```python
from build123d import *

# Parameters (mm, degrees)
F1_DEPTH = 30
F2_R     = 3
F3_DEPTH = 60.001
F5_DEPTH = 30.001


with BuildPart() as f1:
    # F0 (on Front) → F1 (new body)
    with BuildSketch(Plane.XZ):
        Polygon((0, 30), (0, 0), (60, 0), (60, 3), (3, 3), (3, 30), align=None)
    extrude(amount=F1_DEPTH)

    # F2 (on face) → F3 (cut, through all)
    with BuildSketch(Plane(origin=(0, 0, 0), x_dir=(0, -1, 0), z_dir=(-1, 0, 0))):
        with Locations((15, 15)):
            Circle(F2_R)
    extrude(amount=-F3_DEPTH, mode=Mode.SUBTRACT)

    # F4 (on face) → F5 (cut, through all)
    with BuildSketch(Plane(origin=(0, 0, 0), x_dir=(1, 0, 0), z_dir=(0, 0, -1))):
        with BuildLine():
            Line((52, 18), (48.109772, 18))
            ThreePointArc((48.109772, 18), (38, 15), (48.109772, 12))
            Line((48.109772, 12), (52, 12))
            ThreePointArc((52, 12), (55, 15), (52, 18))
        make_face()
    extrude(amount=-F5_DEPTH, mode=Mode.SUBTRACT)


solid = f1.part
```
Input: part model. Units: mm. Frame: model coordinates. A direction names the side the tool comes from. Round coordinates to 2 decimals unless told otherwise and drop trailing zeros. Loops run counter-clockwise (first coordinate to the right, second up) from the corner with the lowest first, then second, coordinate; pieces in that order, holes last. Notation, with made-up numbers: (74.25, 23.5) -> (90.25, 23.5) arc R12 ccw to (90.25, 28.5) -> close; hole circle Ø10 at (64, 65). An arc over 180 degrees is marked (long way). Use one line per item in the form item = value. Start each with the question number.
Item 1: Section query C-C on x = 43.5. Return the cut outline in (y, z), then the cut area to 3 significant figures.
Item 2: Section query D-D on y = -10.75. Return the cut outline in (x, z), then the cut area to 3 significant figures.
Item 3: Contact query for a flat-ended pin moving along its axis: pin 1 Ø1.5 at (x, y) = (28, -11.5) entering from +Z. Output: stop coordinate, or through.
Item 4: Section query B-B on y = -15. Return the cut outline in (x, z), then the cut area to 3 significant figures.
Item 5: Mould query, pull axis Y, two halves, no side actions, for faces 4 (the face through (23.2, 0, 2.8)), 5 (the face through (50, -18, 1)), 6 (the face through (32, -15, 3)). Classes: pulls with the +Y half, pulls with the -Y half, needs draft (parallel to the pull), parting line crosses it, or undercut.
Item 6: Section query A-A on z = 15. Return the cut outline in (x, y), then the cut area to 3 significant figures.
Item 7: Set-up query: faces 1 (the face through (0, -15, 19)), 2 (the face through (3, -15, 19)), 3 (the face through (55, -15, 1)). Return all of +Z, -Z, +X, -X, +Y, -Y with unobstructed straight access to the full face (end or side cutting, diameter ignored); none if empty.
Item 8: Material intervals for L1, parallel to Y at x = 43.5, z = 1.85; L2, parallel to X at y = -15, z = 0.7; L3, parallel to Z at x = 25.5, y = -7, sorted ascending. Write a range as from..to.
Ans:
q1.outline = (-30, 0) -> (-20.5, 0) -> (-20.5, 3) -> (-30, 3) -> close; (-9.5, 0) -> (0, 0) -> (0, 3) -> (-9.5, 3) -> close
q1.area = 57.0 mm^2
q2.outline = (0, 0) -> (40.01, 0) -> (40.01, 3) -> (3, 3) -> (3, 30) -> (0, 30) -> close; (46.99, 0) -> (60, 0) -> (60, 3) -> (46.99, 3) -> close
q2.area = 240 mm^2
q3.pin_1 = 3
q4.outline = (0, 0) -> (38, 0) -> (38, 3) -> (3, 3) -> (3, 12) -> (0, 12) -> close; (0, 18) -> (3, 18) -> (3, 30) -> (0, 30) -> close; (55, 0) -> (60, 0) -> (60, 3) -> (55, 3) -> close
q4.area = 192 mm^2
q5.face_4 = pulls with the +Y half
q5.face_5 = undercut
q5.face_6 = needs draft
q6.outline = (0, -30) -> (3, -30) -> (3, -18) -> (0, -18) -> close; (0, -12) -> (3, -12) -> (3, 0) -> (0, 0) -> close
q6.area = 72.0 mm^2
q7.face_1 = +Z, -Z, -X, +Y, -Y
q7.face_2 = +Z, +X, +Y, -Y
q7.face_3 = +Z, -Z
q8.L1 = -30..-20.5, -9.5..0
q8.L2 = 0..38, 55..60
q8.L3 = 0..3
